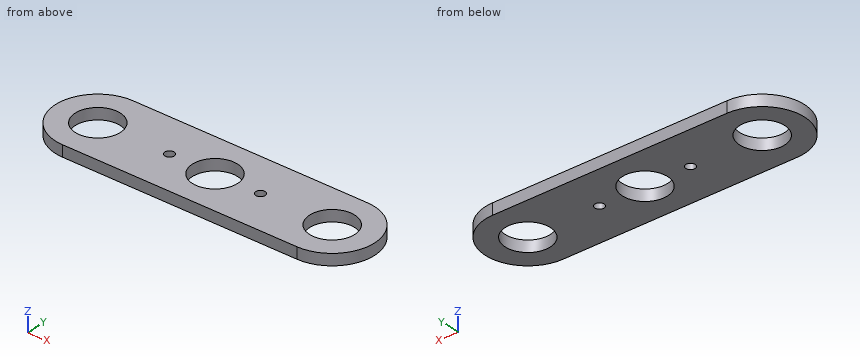
from build123d import *

# Parameters (mm, degrees)
SKETCH2_R           = 11.99
BOSS_EXTRUDE1_DEPTH = 6
SKETCH3_R           = 2.5
CUT_EXTRUDE1_DEPTH  = 10


with BuildPart() as part:
    # Sketch2 → Boss-Extrude1 (new body)
    with BuildSketch(Plane.XY):
        with BuildLine():
            Line((-62.5, -22.5), (62.5, -22.5))
            ThreePointArc((62.5, -22.5), (85, 0), (62.5, 22.5))
            Line((62.5, 22.5), (-62.5, 22.5))
            ThreePointArc((-62.5, 22.5), (-85, 0), (-62.5, -22.5))
        make_face()
        with Locations((-62.5, 0)):
            Circle(SKETCH2_R, mode=Mode.SUBTRACT)
        with Locations(Location((62.5, 0, 0), (0, 0, 180))):
            Circle(SKETCH2_R, mode=Mode.SUBTRACT)
        Circle(SKETCH2_R, mode=Mode.SUBTRACT)
    extrude(amount=BOSS_EXTRUDE1_DEPTH)

    # Sketch3 → Cut-Extrude1 (cut)
    with BuildSketch(Plane.XY.offset(6)):
        with Locations((-24.25, 0)):
            Circle(SKETCH3_R)
        with Locations((24.25, 0)):
            Circle(SKETCH3_R)
    extrude(amount=-CUT_EXTRUDE1_DEPTH, mode=Mode.SUBTRACT)


solid = part.part
Here's how the part is built. I have some questions about the finished solid (model axes, mm). Round coordinates to 2 decimals unless told otherwise and drop trailing zeros. Order: outer loops, then holes, each group sorted by start corner. A loop starts at its lowest first (then second) coordinate and runs counter-clockwise, first axis right, second up. Notation, with made-up numbers: (83, 86) -> (91, 86) arc R23 cw to (91, 101) -> close; hole circle Ø6 at (-35.5, 77). An arc over 180 degrees is marked (long way). Return JSON: item names as keys, results as strings.
Q1. If we section it at B-B on z = 1: List the corners of the cut face in (x, y) for me.
Filled sheet:
{"outline": "(-62.5, -22.5) -> (62.5, -22.5) arc R22.5 ccw to (62.5, 22.5) -> (-62.5, 22.5) arc R22.5 ccw to start; hole circle Ø23.98 at (-62.5, 0); hole circle Ø5 at (-24.25, 0); hole circle Ø23.98 at (0, 0); hole circle Ø5 at (24.25, 0); hole circle Ø23.98 at (62.5, 0)"}
Q2. For pin 1 Ø4 at (x, y) = (-39.5, 14) entering from -Z; pin 2 Ø2 at (y, z) = (7.5, 1) entering from -X, each with a flat end and sliding along its axis, tell me the tip position at first contact or that it passes through.
Filled sheet:
{"pin 1": "stops at z = 0", "pin 2": "stops at x = -84.04"}
Q3. I need wall thicknesses on line 1 along Y through (x, z) = (-62.5, 2.8); line 2 along Y through (x, z) = (-24.25, 2.1); line 3 along X through (y, z) = (-3, 2.7). Which ranges of each line are inside material? Lowest first, please. Write a range as from..to.
Filled sheet:
{"line 1": "y = -22.5..-11.99, 11.99..22.5", "line 2": "y = -22.5..-2.5, 2.5..22.5", "line 3": "x = -84.8..-74.11, -50.89..-11.61, 11.61..50.89, 74.11..84.8"}
Q4. If we section it at D-D on y = -9: List the corners of the cut face in (x, z) for me, plus the area to 3 significant figures.
Filled sheet:
{"outline": "(-83.12, 0) -> (-70.42, 0) -> (-70.42, 6) -> (-83.12, 6) -> close; (-54.58, 0) -> (-7.92, 0) -> (-7.92, 6) -> (-54.58, 6) -> close; (7.92, 0) -> (54.58, 0) -> (54.58, 6) -> (7.92, 6) -> close; (70.42, 0) -> (83.12, 0) -> (83.12, 6) -> (70.42, 6) -> close", "area": "712 mm^2"}
Q5. If we section it at C-C on y = 0: List the corners of the cut face in (x, z) for me, plus the area to 3 significant figures.
Filled sheet:
{"outline": "(-85, 0) -> (-74.49, 0) -> (-74.49, 6) -> (-85, 6) -> close; (-50.51, 0) -> (-26.75, 0) -> (-26.75, 6) -> (-50.51, 6) -> close; (-21.75, 0) -> (-11.99, 0) -> (-11.99, 6) -> (-21.75, 6) -> close; (11.99, 0) -> (21.75, 0) -> (21.75, 6) -> (11.99, 6) -> close; (26.75, 0) -> (50.51, 0) -> (50.51, 6) -> (26.75, 6) -> close; (74.49, 0) -> (85, 0) -> (85, 6) -> (74.49, 6) -> close", "area": "528 mm^2"}
Q6. If we section it at A-A on x = 0: List the corners of the cut face in (y, z) for me.
Filled sheet:
{"outline": "(-22.5, 0) -> (-11.99, 0) -> (-11.99, 6) -> (-22.5, 6) -> close; (11.99, 0) -> (22.5, 0) -> (22.5, 6) -> (11.99, 6) -> close"}
